Autodesk Inventor part; units mm, degrees
ref_plane "YZ Plane" through (0, 0, 0) normal (1, 0, 0) x (0, 1, 0)
ref_plane "XZ Plane" through (0, 0, 0) normal (0, 1, 0) x (-1, 0, 0)
ref_plane "XY Plane" through (0, 0, 0) normal (0, 0, 1) x (1, 0, 0)
sketch "Sketch1" plane through (0, 0, 0) normal (0, 1, 0) x (-1, 0, 0)
  line L0 (10.75, 7) -> (-10.75, 7)
  line L1 (-10.75, 7) -> (-10.75, -7)
  line L2 (-10.75, -7) -> (10.75, -7)
  line L3 (10.75, -7) -> (10.75, 7)
  point P0 (0, 0)
  dimension "d0" = 21.5
  dimension "d1" = 14
  dimension "d2" = 10.75
  dimension "d3" = 7
extrude "Extrusion1" add sketch "Sketch1" along normal blind 5
sketch "Sketch2" plane through (0, 5, 0) normal (0, 1, 0) x (1, 0, 0)
  circle A0 centre (3.75, 0) radius 5
  line L0 (10.75, 7) -> (-10.75, 7)
  line L1 (10.75, -7) -> (10.75, 7)
  point P0 (0, 0)
  dimension "d6" = 10
  dimension "d7" = 7
  dimension "d8" = 7
extrude "Extrusion2" add sketch "Sketch2" along normal blind 1
fillet "Fillet1" radius 2 1 edges at (-1.25, 5, 0)
fillet "Fillet2" radius 1 4 edges at (10.75, 2.5, 7) (10.75, 2.5, -7) (-10.75, 2.5, 7) (-10.75, 2.5, -7)
fillet "Fillet3" radius 0.5 9 edges at (-1.25, 6, 0) (10.4571, 5, 6.7071) (10.75, 5, 0) (10.4571, 5, -6.7071) (0, 5, -7) (-10.4571, 5, -6.7071) (-10.75, 5, 0) (-10.4571, 5, 6.7071) (0, 5, 7)
sketch "Sketch3" plane through (0, 0, 0) normal (0, -1, 0) x (1, 0, 0)
  line L0 (-6, 3) -> (6, 3)
  line L1 (6, 3) -> (6, -3)
  line L2 (6, -3) -> (-6, -3)
  line L3 (-6, -3) -> (-6, 3)
  line L4 (-9.75, 7) -> (9.75, 7)
  point P0 (0, 0)
  dimension "d14" = 12
  dimension "d15" = 6
  dimension "d16" = 4
  dimension "d17" = 6
extrude "Extrusion3" cut sketch "Sketch3" against normal blind 4.5
properties part number "Black_Keyboard_Button"
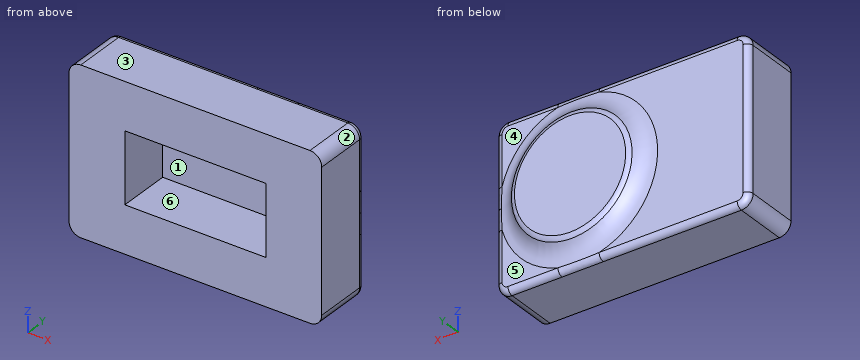
For this review, take the finished solid that the model builds, in its own axes (mm). Face numbers are marked on the shaded views. A direction names the side the tool comes from. Coordinates: 2 decimals unless noted, no trailing zeros. Order: outer loops, then holes, each group sorted by start corner. A loop starts at its lowest first (then second) coordinate and runs counter-clockwise, first axis right, second up. Notation, with made-up numbers: (76.5, 31.25) -> (99.5, 31.25) arc R14 cw to (99.5, 50.25) -> close; hole circle Ø2 at (70.5, 65.25). An arc over 180 degrees is marked (long way). Use CSV: the item, a comma, the result in double quotes. Start each with the question number.
Item 1: We need section B-B, the plane x = -3.5. Give the boundary of the cut face in (y, z).
Item 2: For the marked faces 4, 5 and 6, list the 3-axis set-ups (+Z, -Z, +X, -X, +Y, -Y) from which the entire face can be reached by the end or side of a thin tool; tool diameter is ignored.
Item 3: We need section C-C, the plane x = -8.5. Give the boundary of the cut face in (y, z).
Item 4: Draft analysis for pull direction X (two halves, no side actions). For the marked faces 1, 2 and 3, state which applies: pulls with the +X half, pulls with the -X half, needs draft (parallel to the pull), parting line crosses it, or undercut.
Item 5: Insertion check: pin 1 (4 mm diameter, centred on x = -1, z = -3, fed in from +Y); pin 2 (1.4 mm diameter, centred on x = 8, z = -5, fed in from +Y); pin 3 (1.8 mm diameter, centred on x = 1.5, z = 0, fed in from -Y); pin 4 (1 mm diameter, centred on x = -6.5, z = 1, fed in from +Y). Each pin has a flat end and moves straight along its axis. Give the tip position at first contact, or say it passes through.
Item 6: We need section A-A, the plane y = 2.75. Give the boundary of the cut face in (x, z).
Item 7: Wall thickness on probe 1 along Z at (x, y) = (0, 4.25); probe 2 along X at (y, z) = (2.75, 0.5); probe 3 along Y at (x, z) = (-4.25, -2.75): over which ranges is each line inside the solid? List them lowest first.
Derived:
1,outline,"(0, -7) -> (4.5, -7) arc R0.5 ccw to (5, -6.5) -> (5, 6.5) arc R0.5 ccw to (4.5, 7) -> (0, 7) -> (0, 3) -> (4.5, 3) -> (4.5, -3) -> (0, -3) -> close"
2,face 4,"+Z, +X, +Y"
2,face 5,"-Z, +X, +Y"
2,face 6,"-Y"
3,outline,"(0, -7) -> (4.5, -7) arc R0.5 ccw to (5, -6.5) -> (5, 6.5) arc R0.5 ccw to (4.5, 7) -> (0, 7) -> close"
4,face 1,"undercut"
4,face 2,"pulls with the +X half"
4,face 3,"needs draft"
5,pin 1,"stops at y = 6"
5,pin 2,"stops at y = 5.2"
5,pin 3,"stops at y = 4.5"
5,pin 4,"stops at y = 5"
6,outline,"(-10.75, -6) arc R1 ccw to (-9.75, -7) -> (9.75, -7) arc R1 ccw to (10.75, -6) -> (10.75, 6) arc R1 ccw to (9.75, 7) -> (-9.75, 7) arc R1 ccw to (-10.75, 6) -> close; hole (-6, -3) -> (6, -3) -> (6, 3) -> (-6, 3) -> close"
7,probe 1,"z = -7 to -3, 3 to 7"
7,probe 2,"x = -10.75 to -6, 6 to 10.75"
7,probe 3,"y = 4.5 to 5"
